Design review of the part shown in the three views and the two pictorial views. Dimensions are in mm from the part's minimum x, y and z. A direction names the side the tool comes from. Give positions to 0.01 mm unless a question says otherwise; leave off trailing zeros. Order: outer loops, then holes, each group sorted by start corner. A loop starts at its lowest first (then second) coordinate and runs counter-clockwise, first axis right, second up.
Item 1: Machinability: for the marked faces 1, 2, 3 and 4, which of the approach directions +Z, -Z, +X, -X, +Y, -Y give a long, thin tool a straight path to every point of the face, cutting with its end or side? Answer none if there is none.
Item 2: Consider section A-A (x = 17.5). Give the boundary of the cut face in (y, z).
Item 3: Consider section B-B (y = 10). Give the boundary of the cut face in (x, z), plus the area to 3 significant figures.
Item 4: For probe 1 along Z at (x, y) = (36, 12.5); probe 2 along X at (y, z) = (17.75, 31.5); probe 3 along Z at (x, y) = (22, 14.5), list the stretches that pass through material, from the lowest coordinate up.
Item 5: Consider section C-C (z = 7.5). Give the boundary of the cut face in (x, y), plus the area to 3 significant figures.
Item 6: For P1, Ø10, axis at y = 13, z = 17, coming from the -X side; P2, Ø2, axis at x = 53, y = 13, coming from the -Z side; P3, Ø4, axis at x = 2, y = 7.5, coming from the +Z side, all flat-tipped, find the tip position at first contact; note any pin that passes through.
Item 7: Consider section D-D (y = 17.5). Give the boundary of the cut face in (x, z).
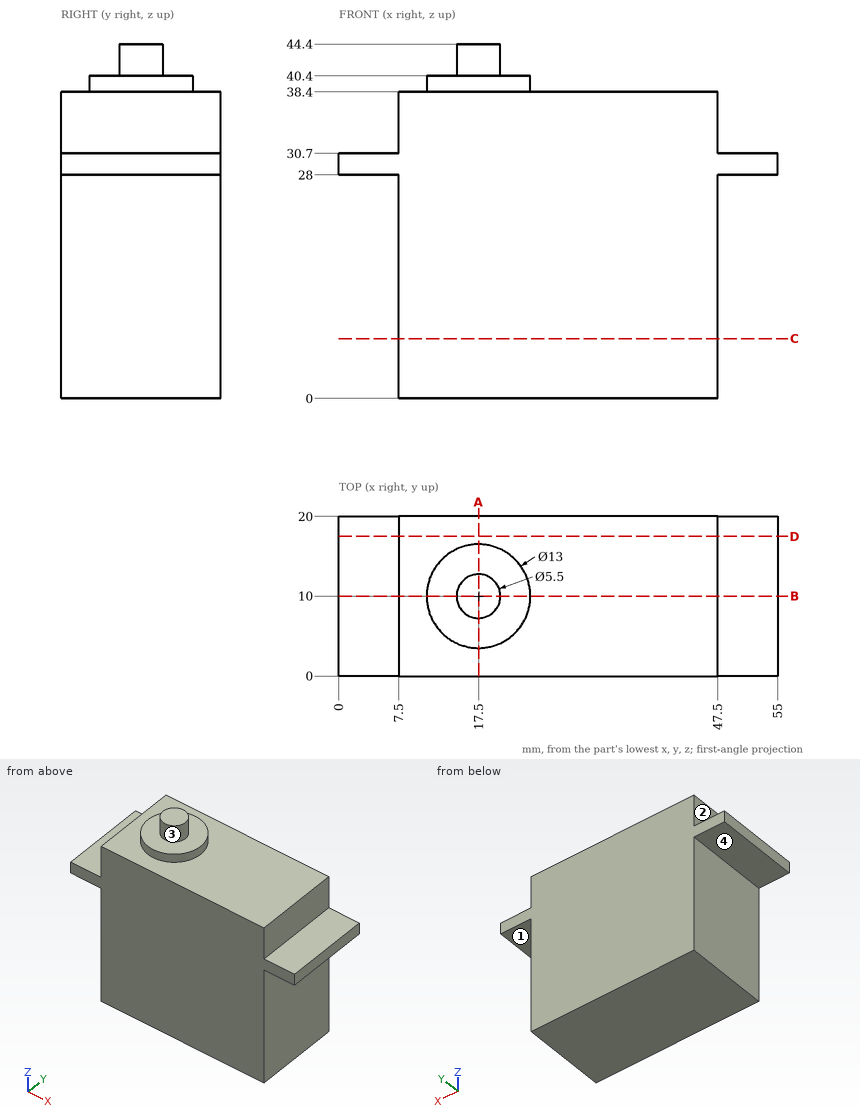
Resolved:
1. face 1: -Z, +X, +Y, -Y
1. face 2: +Z, -X, +Y, -Y
1. face 3: +Z
1. face 4: -Z, -X, +Y, -Y
2. outline: (0, 0) - (20, 0) - (20, 38.4) - (16.5, 38.4) - (16.5, 40.4) - (12.75, 40.4) - (12.75, 44.4) - (7.25, 44.4) - (7.25, 40.4) - (3.5, 40.4) - (3.5, 38.4) - (0, 38.4) - close
3. outline: (0, 28) - (7.5, 28) - (7.5, 0) - (47.5, 0) - (47.5, 28) - (55, 28) - (55, 30.7) - (47.5, 30.7) - (47.5, 38.4) - (24, 38.4) - (24, 40.4) - (20.25, 40.4) - (20.25, 44.4) - (14.75, 44.4) - (14.75, 40.4) - (11, 40.4) - (11, 38.4) - (7.5, 38.4) - (7.5, 30.7) - (0, 30.7) - close
3. area: 1,620 mm2
4. probe 1: z = 0 to 38.4
4. probe 2: x = 7.5 to 47.5
4. probe 3: z = 0 to 40.4
5. outline: (7.5, 0) - (47.5, 0) - (47.5, 20) - (7.5, 20) - close
5. area: 800 mm2
6. P1: stops at x = 7.5
6. P2: stops at z = 28
6. P3: stops at z = 30.7
7. outline: (0, 28) - (7.5, 28) - (7.5, 0) - (47.5, 0) - (47.5, 28) - (55, 28) - (55, 30.7) - (47.5, 30.7) - (47.5, 38.4) - (7.5, 38.4) - (7.5, 30.7) - (0, 30.7) - close
